Design review of the part built by this model. Coordinates are the model's own, in mm. Give positions to 0.01 mm unless a question says otherwise; leave off trailing zeros. Write each loop counter-clockwise with the first axis right and the second up, starting at its lowest first coordinate (ties: lowest second). Pieces come first, ordered by that corner, then holes. Notation, with made-up numbers: (44.5, 77.25) -> (96.5, 77.25) arc R16 cw to (96.5, 88.25) -> close; hole circle Ø4 at (-31, 64.5). An arc over 180 degrees is marked (long way). Use CSV: the item, a comma, the result in double quotes.
```python
from build123d import *

# Parameters (mm, degrees)
BOSS_EXTRUDE1_DEPTH = 20
SKETCH1_3_R         = 5
BOSS_EXTRUDE2_DEPTH = 120
SKETCH4_W           = 2
SKETCH4_H           = 2.701125373


with BuildPart() as part:
    # Sketch1 → Boss-Extrude1 (new body)
    with BuildSketch(Plane.XY):
        with BuildLine():
            Line((2, 2.5), (0, 2.5))
            Line((0, 2.5), (-2, 2.5))
            Line((-2, 2.5), (-2, 4.582575695))
            ThreePointArc((-2, 4.582575695), (-2.738612788, -4.183300133), (5, 0))
            ThreePointArc((5, 0), (4.183300133, 2.738612788), (2, 4.582575695))
            Line((2, 4.582575695), (2, 2.5))
        make_face()
    extrude(amount=BOSS_EXTRUDE1_DEPTH)

    # Sketch1_3 → Boss-Extrude2 (add)
    with BuildSketch(Plane.XY):
        Circle(SKETCH1_3_R)
    extrude(amount=-BOSS_EXTRUDE2_DEPTH)

    # Sketch4 → Cut-Revolve2 (revolve, cut)
    with BuildSketch(Plane.XY):
        with Locations((1, 3.850562686)):
            Rectangle(SKETCH4_W, SKETCH4_H)
    revolve(axis=Axis((0, 0, 0), (0, 1, 0)), mode=Mode.SUBTRACT)


solid = part.part
```
(1) Mouldability with a two-part tool opening along X and no side actions: class faces 1 (the face through (0, 2.5, 9)), 2 (the face through (0, 4, -2)), 3 (the face through (0, 0, -120)) as +X half, -X half, draft (parallel to the pull), parting line (faces both ways), or undercut.
Established:
face 1,"undercut"
face 2,"undercut"
face 3,"draft"
(2) For line 1 along X through (y, z) = (0.25, 5); line 2 along X through (y, z) = (4.5, 5); line 3 along Y through (x, z) = (-3.5, -83), list the stretches that pass through material, from the lowest coordinate up. Write a range as [from, to].
Established:
line 1,"x = [-4.99, 4.99]"
line 2,"x = [-2.18, -2], [2, 2.18]"
line 3,"y = [-3.57, 3.57]"
(3) Take a section at A-A (x = 0). Write out the cut boundary in (y, z).
Established:
outline,"(-5, -120) -> (5, -120) -> (5, -2) -> (2.5, -2) -> (2.5, 20) -> (-5, 20) -> close"
(4) Clearance check with flat-ended pins moving along their axes: pin 1 (1 mm diameter, centred on x = 3.5, z = -22.5, fed in from -Y); pin 2 (1 mm diameter, centred on y = 4, z = 10, fed in from +X); pin 3 (1.7 mm diameter, centred on y = 4, z = 10, fed in from -X); pin 4 (5 mm diameter, centred on y = 2, z = -44, fed in from +X). State where each tip first meets the part, or that it passes through.
Established:
pin 1,"stops at y = -4"
pin 2,"stops at x = 3.57"
pin 3,"stops at x = -3.88"
pin 4,"stops at x = 5"
(5) Take a section at C-C (z = -59). Write out the cut boundary in (x, y).
Established:
outline,"circle Ø10 at (0, 0)"
(6) Take a section at B-B (y = -3). Write out the cut boundary in (x, z), then the cut area to 3 significant figures.
Established:
outline,"(-4, -120) -> (4, -120) -> (4, 20) -> (-4, 20) -> close"
area,"1,120 mm2"
